Input: part model. Units: mm. Frame: model coordinates. Coordinates: 2 decimals unless noted, no trailing zeros. Order: outer loops, then holes, each group sorted by start corner. A loop starts at its lowest first (then second) coordinate and runs counter-clockwise, first axis right, second up. Notation, with made-up numbers: M 20.5,53 L 73.5,53 A25 cw 73.5,81 Z; hole C 7.25,81.25 d1. An arc over 180 degrees is marked long. One line per item, written item: value.
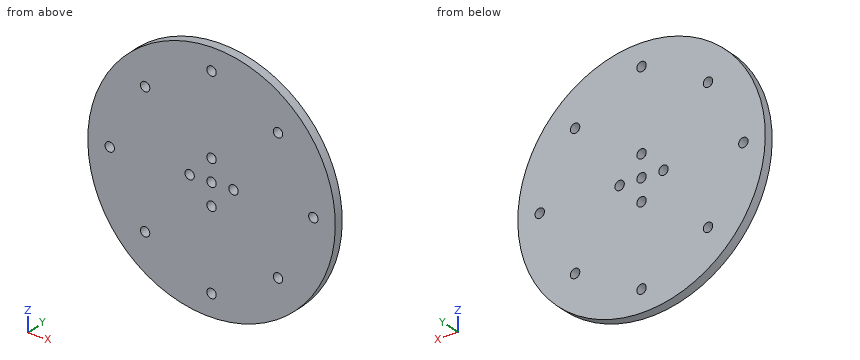
```python
from build123d import *

# Parameters (mm, degrees)
SKETCH_1_R               = 39.5
SKETCH_1_R_2             = 1.5
EXTRUDE_1_DEPTH          = 3
CUT_EXTRUDE_1_DEPTH      = 56.941934182
CUT_EXTRUDE_1_DEPTH_BACK = 56.941934182
SKETCH_2_R               = 1.5


with BuildPart() as part:
    # 草图1 → 凸台-拉伸1 (new body)
    with BuildSketch(Plane(origin=(0, 0, 0), x_dir=(1, 0, 0), z_dir=(0, 1, 0))):
        with Locations(Location((0, 0, 0), (0, 0, 270))):
            Circle(SKETCH_1_R)
        with Locations(Location((0, 32.5, 0), (0, 0, 270))):
            Circle(SKETCH_1_R_2, mode=Mode.SUBTRACT)
        with Locations(Location((32.5, 0, 0), (0, 0, 270))):
            Circle(SKETCH_1_R_2, mode=Mode.SUBTRACT)
        with Locations(Location((0, -32.5, 0), (0, 0, 270))):
            Circle(SKETCH_1_R_2, mode=Mode.SUBTRACT)
        with Locations(Location((-32.5, 0, 0), (0, 0, 270))):
            Circle(SKETCH_1_R_2, mode=Mode.SUBTRACT)
        with Locations(Location((21.213203436, 21.213203436, 0), (0, 0, 270))):
            Circle(SKETCH_1_R_2, mode=Mode.SUBTRACT)
        with Locations(Location((21.213203436, -21.213203436, 0), (0, 0, 270))):
            Circle(SKETCH_1_R_2, mode=Mode.SUBTRACT)
        with Locations(Location((-21.213203436, -21.213203436, 0), (0, 0, 270))):
            Circle(SKETCH_1_R_2, mode=Mode.SUBTRACT)
        with Locations(Location((-21.213203436, 21.213203436, 0), (0, 0, 270))):
            Circle(SKETCH_1_R_2, mode=Mode.SUBTRACT)
    extrude(amount=EXTRUDE_1_DEPTH)

    # 草图2 → 切除-拉伸1 (cut, two sides: drawn at the far end of the back side and taken through both)
    with BuildSketch(Plane(origin=(0, 3, 0), x_dir=(1, 0, 0), z_dir=(0, 1, 0)).offset(-CUT_EXTRUDE_1_DEPTH_BACK)):
        with Locations(Location((0, 0, 0), (0, 0, 270))):
            Circle(SKETCH_2_R)
        with Locations(Location((0, 7, 0), (0, 0, 270))):
            Circle(SKETCH_2_R)
        with Locations(Location((7, 0, 0), (0, 0, 270))):
            Circle(SKETCH_2_R)
        with Locations(Location((0, -7, 0), (0, 0, 270))):
            Circle(SKETCH_2_R)
        with Locations(Location((-7, 0, 0), (0, 0, 270))):
            Circle(SKETCH_2_R)
    extrude(amount=CUT_EXTRUDE_1_DEPTH + CUT_EXTRUDE_1_DEPTH_BACK, mode=Mode.SUBTRACT)


solid = part.part
```
(1) Cut plane A-A on z = 0. Output: boundary loops of the cut face in (x, y).
Data:
outline: M -39.5,0 L -34,0 L -34,3 L -39.5,3 Z; M -31,0 L -8.5,0 L -8.5,3 L -31,3 Z; M -5.5,0 L -1.5,0 L -1.5,3 L -5.5,3 Z; M 1.5,0 L 5.5,0 L 5.5,3 L 1.5,3 Z; M 8.5,0 L 31,0 L 31,3 L 8.5,3 Z; M 34,0 L 39.5,0 L 39.5,3 L 34,3 Z
(2) Ray query, line 1 (X direction, y = 1.8, z = 0); line 2 (X direction, y = 0.2, z = -21); line 3 (Z direction, x = 0.5, y = 2.8). Return the intervals inside material, ascending. Write a range as from..to.
Data:
line 1: x = -39.5..-34, -31..-8.5, -5.5..-1.5, 1.5..5.5, 8.5..31, 34..39.5
line 2: x = -33.46..-22.7, -19.73..19.73, 22.7..33.46
line 3: z = -39.5..-33.91, -31.09..-8.41, -5.59..-1.41, 1.41..5.59, 8.41..31.09, 33.91..39.5
(3) Cut plane C-C on z = 32.5. Output: boundary loops of the cut face in (x, y), plus the area to 3 significant figures.
Data:
outline: M -22.45,0 L -1.5,0 L -1.5,3 L -22.45,3 Z; M 1.5,0 L 22.45,0 L 22.45,3 L 1.5,3 Z
area: 126 mm2
(4) Cut plane B-B on y = 0.75. Give the number of separate pieces and of enclosed holes in the cut face, plus the area to 3 significant figures.
Data:
separate pieces: 1
enclosed holes: 13
area: 4,810 mm2
(5) First-contact query: pin 1 (1.8 mm diameter, centred on x = -7, z = 0, fed in from -Y); pin 2 (1 mm diameter, centred on x = -30.5, y = 0.5, fed in from -Z). Flat tips, straight axial feed; report the tip coordinate or a pass-through.
Data:
pin 1: passes through
pin 2: stops at z = -25.7
(6) Cut plane D-D on x = 32.5. Output: boundary loops of the cut face in (y, z), plus the area to 3 significant figures.
Data:
outline: M 0,-22.45 L 3,-22.45 L 3,-1.5 L 0,-1.5 Z; M 0,1.5 L 3,1.5 L 3,22.45 L 0,22.45 Z
area: 126 mm2
